Geometry: final body of the model. Coordinates: model frame, mm. A direction names the side the tool comes from. Round coordinates to 2 decimals unless told otherwise and drop trailing zeros. Loops run counter-clockwise (first coordinate to the right, second up) from the corner with the lowest first, then second, coordinate; pieces in that order, holes last. Notation, with made-up numbers: (-11.75, -39) - (26.25, -39) arc R12 cw to (26.25, -22) - close; hole circle Ø2 at (2, -29.75). An arc over 180 degrees is marked (long way). Answer as a JSON object with one key per item and string values. Group by question number.
Item 1: First-contact query: pin 1 (5 mm diameter, centred on y = 9, z = -4.5, fed in from +X); pin 2 (4 mm diameter, centred on x = 18, y = 16, fed in from +Z); pin 3 (5 mm diameter, centred on y = 14, z = -7, fed in from -X). Flat tips, straight axial feed; report the tip coordinate or a pass-through.
Item 2: Line query: line 1 (X direction, y = 6.75, z = -2); line 2 (X direction, y = 2.5, z = -6.75); line 3 (Z direction, x = 13.75, y = 7.5). Output: solid intervals per line, ascending.
Item 3: Section D-D (x = 10.5). Return the cut outline in (y, z).
Item 4: Reachability of faces 1 (the face through (2, 12, -1.5)), 2 (the face through (0, 9, -7)), 3 (the face through (4.6, 9, -7)) from +Z, -Z, +X, -X, +Y, -Y: full face, straight path, thin tool, end or side. Return the list, or none.
Item 5: Draft query along Z for faces 4 (the face through (2, 12, -11.6)), 5 (the face through (10, 9, -15)), 6 (the face through (2, 9, 0)). Return one class per face: released by +Z, released by -Z, zero draft, split by the parting line, or undercut.
Item 6: Section C-C (z = -6). Return the cut outline in (x, y), plus the area to 3 significant figures.
Item 7: Section A-A (y = 12.5). Return the cut outline in (x, z).
Item 8: Section B-B (y = 1.25). Return the cut outline in (x, z), plus the area to 3 significant figures.
```python
from build123d import *

# Parameters (mm, degrees)
BOSS_EXTRUDE1_DEPTH = 4.5
SKETCH1_3_W         = 1.65
SKETCH1_3_H         = 10.1
BOSS_EXTRUDE2_DEPTH = 19


with BuildPart() as part:
    # Sketch1 → Boss-Extrude1 (new body)
    with BuildSketch(Plane(origin=(0, 0, 0), x_dir=(1, 0, 0), z_dir=(0, 1, 0))):
        Polygon((0, 0), (0, 15), (20, 15), (20, 13.5), (4.6, 13.5), (4.6, 0), align=None)
    extrude(amount=BOSS_EXTRUDE1_DEPTH)

    # Sketch1<3> → Boss-Extrude2 (add)
    with BuildSketch(Plane(origin=(0, 0, 0), x_dir=(1, 0, 0), z_dir=(0, 1, 0))):
        Polygon((0, 0), (0, 15), (20, 15), (20, 13.5), (4.6, 13.5), (4.6, 0), align=None)
        with Locations((2.325, 6.55)):
            Rectangle(SKETCH1_3_W, SKETCH1_3_H, mode=Mode.SUBTRACT)
    extrude(amount=BOSS_EXTRUDE2_DEPTH)


solid = part.part
```
Values:
{
 "1": {"pin 1": "stops at x = 4.6", "pin 2": "stops at z = -13.5", "pin 3": "stops at x = 0"},
 "2": {"line 1": "x = 0 to 1.5, 3.15 to 4.6", "line 2": "x = 0 to 4.6", "line 3": "z = -15 to -13.5"},
 "3": {"outline": "(0, -15) - (19, -15) - (19, -13.5) - (0, -13.5) - close"},
 "4": {"face 1": "+Y", "face 2": "+Z, -Z, -X, +Y, -Y", "face 3": "+Z, +X, +Y, -Y"},
 "5": {"face 4": "undercut", "face 5": "released by -Z", "face 6": "released by +Z"},
 "6": {"outline": "(0, 0) - (4.6, 0) - (4.6, 19) - (3.15, 19) - (3.15, 4.5) - (1.5, 4.5) - (1.5, 19) - (0, 19) - close", "area": "63.5 mm^2"},
 "7": {"outline": "(0, -15) - (20, -15) - (20, -13.5) - (4.6, -13.5) - (4.6, 0) - (0, 0) - close; hole (1.5, -11.6) - (3.15, -11.6) - (3.15, -1.5) - (1.5, -1.5) - close"},
 "8": {"outline": "(0, -15) - (20, -15) - (20, -13.5) - (4.6, -13.5) - (4.6, 0) - (0, 0) - close", "area": "92.1 mm^2"}
}
